The model under review builds one solid part; all positions refer to its coordinate system, in mm. A direction names the side the tool comes from. Coordinates: 2 decimals unless noted, no trailing zeros. Order: outer loops, then holes, each group sorted by start corner. A loop starts at its lowest first (then second) coordinate and runs counter-clockwise, first axis right, second up. Notation, with made-up numbers: (19, 42.5) -> (66, 42.5) arc R21 ccw to (66, 53.5) -> close; hole circle Ø3 at (23.25, 26). An arc over 180 degrees is marked (long way). Use one line per item in the form item = value. Start each with the question number.
(1) Take a section at A-A (z = 6). State the section outline as (x, y) points (3 decimals).
(2) For faces 1 (the flat face through (41.275, -1, 4)), 2 (the flat face through (1, 35, 9.525)), 3 (the flat face through (46, -25.4, 42)), list the 3-axis set-ups (+Z, -Z, +X, -X, +Y, -Y) from which the entire face can be reached by the end or side of a thin tool; tool diameter is ignored.
(3) Take a section at B-B (y = 40). State the section outline as (x, z) points (3 decimals).
(4) Wall thickness on line 1 along Z through (x, y) = (41, -31) (3 decimals); line 2 along Y through (x, z) = (80.5, 45.5); line 3 along Y through (x, z) = (40, 59): over which ranges is each line inside the solid? List them lowest first.
(5) Mouldability with a two-part tool opening along X and no side actions: class faces 4 (the cylindrical face through (32.13, 16.55, 51.37)), 5 (the flat face through (-1, -1, -9.525)), 6 (the cylindrical face through (39.464, -61.59, 0.133)), 7 (the cylindrical face through (45.8, -0.4, 38.1)) as +X half, -X half, draft (parallel to the pull), parting line (faces both ways), or undercut.
(6) Insertion check: pin 1 Ø11 at (y, z) = (-17, 0.5) entering from +X (3 decimals); pin 2 Ø4 at (x, z) = (93.5, 56.5) entering from -Y; pin 3 Ø10 at (y, z) = (-26, 34) entering from -X. Each pin has a flat end and moves straight along its axis. Give the tip position at first contact, or say it passes through.
```python
from build123d import *

# Parameters (mm, degrees)
F1_DEPTH = 63.5
F2_DEPTH = 25.4
F3_DEPTH = 7.9375
F5_R     = 6.35


with BuildPart() as f1:
    # F0 (on Front) → F1 (new body, symmetric)
    with BuildSketch(Plane.XZ):
        Polygon((22.225, 9.525), (-41.275, 9.525), (-41.275, -9.525), (41.275, -9.525), (41.275, 9.525), align=None)
    extrude(amount=F1_DEPTH, both=True)

    # F0 (on Front) → F2 (join, symmetric)
    with BuildSketch(Plane.XZ):
        with BuildLine():
            Line((22.225, 27.0002), (22.225, 9.525))
            Line((22.225, 9.525), (41.275, 9.525))
            Line((41.275, 9.525), (41.275, 27.0002))
            ThreePointArc((41.275, 27.0002), (45.9246798487, 38.2255201513), (57.15, 42.8752))
            Line((57.15, 42.8752), (60.325, 42.8752))
            Line((60.325, 42.8752), (60.325, 61.9252))
            Line((60.325, 61.9252), (57.15, 61.9252))
            add(Edge.make_bspline(
                [(55.4794704974, 61.8852248127), (56.036011294, 61.9013524911), (56.5928753418, 61.9146861922), (57.15, 61.9252)],
                knots=[110.2645678644, 110.2645678644, 110.2645678644, 110.2645678644, 111.5045361635, 111.5045361635, 111.5045361635, 111.5045361635], degree=3))
            ThreePointArc((55.4794704974, 61.8852248127), (31.8705729112, 51.0980461913), (22.225, 27.0002))
        make_face()
        Polygon((85.7179611921, 61.9252), (60.325, 61.9252), (60.325, 42.8752), (85.723823737, 42.8752), align=None)
    extrude(amount=F2_DEPTH, both=True)

    # F0 (on Front) → F3 (join, symmetric)
    with BuildSketch(Plane.XZ):
        with BuildLine():
            add(Edge.make_bspline(
                [(-41.275, 9.525), (-40.945480422, 36.9229423767), (5.9889065218, 60.4510659796), (55.4794704974, 61.8852248127)],
                knots=[0, 0, 0, 0, 110.2645678644, 110.2645678644, 110.2645678644, 110.2645678644], degree=3))
            Line((-41.275, 9.525), (22.225, 9.525))
            Line((22.225, 9.525), (22.225, 27.0002))
            ThreePointArc((22.225, 27.0002), (31.8705729112, 51.0980461913), (55.4794704974, 61.8852248127))
        make_face()
    extrude(amount=F3_DEPTH, both=True)

    # F0 (on Front) → F4 (revolve)
    with BuildSketch(Plane.XZ):
        Polygon((111.125, 66.675), (85.725, 66.675), (85.7337938173, 38.1), (111.125, 38.1), align=None)
    revolve(axis=Axis((85.7293969086, 0, 52.3875), (0.0003077451, 0, -0.9999999526)))

    # F5
    f5_edges = [f1.edges().sort_by_distance(p)[0] for p in [
        (-41.275, -63.5, 0),
        (41.275, -63.5, 0),
        (41.275, 63.5, 0),
        (-41.275, 63.5, 0),
    ]]
    fillet(f5_edges, radius=F5_R)


solid = f1.part
```
Findings:
q1.outline = (-41.275, -57.15) arc R6.35 ccw to (-34.925, -63.5) -> (34.925, -63.5) arc R6.35 ccw to (41.275, -57.15) -> (41.275, 57.15) arc R6.35 ccw to (34.925, 63.5) -> (-34.925, 63.5) arc R6.35 ccw to (-41.275, 57.15) -> close
q2.face_1 = -Z, +X, +Y, -Y
q2.face_2 = +Z, -X, +Y
q2.face_3 = +Z, +X, -X, -Y
q3.outline = (-41.275, -9.525) -> (41.275, -9.525) -> (41.275, 9.525) -> (-41.275, 9.525) -> close
q4.line_1 = -9.525 to 9.525
q4.line_2 = -25.4 to 25.4
q4.line_3 = -7.94 to 7.94
q5.face_4 = -X half
q5.face_5 = draft
q5.face_6 = +X half
q5.face_7 = undercut
q6.pin_1 = 41.275
q6.pin_2 = -24.73
q6.pin_3 = 22.28
